from build123d import *

# Parameters (mm, degrees)
F0_R     = 2.26
F0_R_2   = 1.98
F1_DEPTH = 3.17
F2_DEPTH = 7.62
F3_SIZE  = 1.8


with BuildPart() as f1:
    # F0 (on Top) → F1 (new body)
    with BuildSketch(Plane.XY):
        with BuildLine():
            Line((0, -32.255), (0, 0))
            Line((0, 0), (0, 32.255))
            Line((0, 32.255), (-30.1, 32.255))
            ThreePointArc((-30.1, 32.255), (-34.342641, 30.497641), (-36.1, 26.255))
            Line((-36.1, 26.255), (-36.1, -26.255))
            ThreePointArc((-36.1, -26.255), (-34.342641, -30.497641), (-30.1, -32.255))
            Line((-30.1, -32.255), (0, -32.255))
        make_face()
        with Locations((-25.91, -22.225)):
            Circle(F0_R, mode=Mode.SUBTRACT)
        with Locations((-20.32, -26.415)):
            Circle(F0_R_2, mode=Mode.SUBTRACT)
        with Locations((-20.32, -15.855)):
            Circle(F0_R_2, mode=Mode.SUBTRACT)
        with Locations((-20.32, -5.295)):
            Circle(F0_R_2, mode=Mode.SUBTRACT)
        with Locations((-25.91, 0)):
            Circle(F0_R, mode=Mode.SUBTRACT)
        with Locations((-20.32, 5.295)):
            Circle(F0_R_2, mode=Mode.SUBTRACT)
        with Locations((-20.32, 15.855)):
            Circle(F0_R_2, mode=Mode.SUBTRACT)
        with Locations((-25.91, 22.225)):
            Circle(F0_R, mode=Mode.SUBTRACT)
        with Locations((-20.32, 26.415)):
            Circle(F0_R_2, mode=Mode.SUBTRACT)
        with BuildLine():
            Line((-30.1, 32.255), (0, 32.255))
            ThreePointArc((0, 32.255), (-0.743949, 34.051051), (-2.54, 34.795))
            Line((-2.54, 34.795), (-11, 34.795))
            Line((-11, 34.795), (-18.1, 36.32))
            Line((-18.1, 36.32), (-30.1752, 36.32))
            ThreePointArc((-30.1752, 36.32), (-35.77888, 33.99888), (-38.1, 28.3952))
            Line((-38.1, 28.3952), (-38.1, 0))
            Line((-38.1, 0), (-38.1, -28.3952))
            ThreePointArc((-38.1, -28.3952), (-35.77888, -33.99888), (-30.1752, -36.32))
            Line((-30.1752, -36.32), (-18.1, -36.32))
            Line((-18.1, -36.32), (-11, -34.795))
            Line((-11, -34.795), (-2.54, -34.795))
            ThreePointArc((-2.54, -34.795), (-0.743949, -34.051051), (0, -32.255))
            Line((0, -32.255), (-30.1, -32.255))
            ThreePointArc((-30.1, -32.255), (-34.342641, -30.497641), (-36.1, -26.255))
            Line((-36.1, -26.255), (-36.1, 26.255))
            ThreePointArc((-36.1, 26.255), (-34.342641, 30.497641), (-30.1, 32.255))
        make_face()
    extrude(amount=F1_DEPTH)

    # F0 (on Top) → F2 (join)
    with BuildSketch(Plane.XY):
        with BuildLine():
            Line((-30.1, 32.255), (0, 32.255))
            ThreePointArc((0, 32.255), (-0.743949, 34.051051), (-2.54, 34.795))
            Line((-2.54, 34.795), (-11, 34.795))
            Line((-11, 34.795), (-18.1, 36.32))
            Line((-18.1, 36.32), (-30.1752, 36.32))
            ThreePointArc((-30.1752, 36.32), (-35.77888, 33.99888), (-38.1, 28.3952))
            Line((-38.1, 28.3952), (-38.1, 0))
            Line((-38.1, 0), (-38.1, -28.3952))
            ThreePointArc((-38.1, -28.3952), (-35.77888, -33.99888), (-30.1752, -36.32))
            Line((-30.1752, -36.32), (-18.1, -36.32))
            Line((-18.1, -36.32), (-11, -34.795))
            Line((-11, -34.795), (-2.54, -34.795))
            ThreePointArc((-2.54, -34.795), (-0.743949, -34.051051), (0, -32.255))
            Line((0, -32.255), (-30.1, -32.255))
            ThreePointArc((-30.1, -32.255), (-34.342641, -30.497641), (-36.1, -26.255))
            Line((-36.1, -26.255), (-36.1, 26.255))
            ThreePointArc((-36.1, 26.255), (-34.342641, 30.497641), (-30.1, 32.255))
        make_face()
    extrude(amount=F2_DEPTH)

    # F3
    f3_edges = [f1.edges().sort_by_distance(p)[0] for p in [
        (-28.17, -22.225, 3.17),
        (-28.17, 0, 3.17),
        (-28.17, 22.225, 3.17),
    ]]
    chamfer(f3_edges, length=F3_SIZE)


solid = f1.part
Verification items for the finished model (mm, model axes). A direction names the side the tool comes from. Give positions to 0.01 mm unless a question says otherwise; leave off trailing zeros. Write each loop counter-clockwise with the first axis right and the second up, starting at its lowest first coordinate (ties: lowest second). Pieces come first, ordered by that corner, then holes.
(1) Material ranges on line 1 (Y direction, x = -25.91, z = 0.3) (3 decimals); line 2 (Y direction, x = -21, z = 5.5) (3 decimals); line 3 (X direction, y = 19.5, z = 7.25), recorded low to high.
(2) Mould release check, pull along X, two halves, no side actions. Record for faces 4 (the face through (-0.724, 34.031, 3.757)), 5 (the face through (-37, 8, 7.62)), 6 (the face through (-18.43, -4.7, 1.56)): +X half, -X half, draft (parallel to the pull), parting line (faces both ways), or undercut.
(3) Cross-section at C-C (x = -20.32). State how many separate pieces and enclosed holes the cut face has, plus the area to 3 significant figures.
(4) Access from +Z, -Z, +X, -X, +Y, -Y to the whole of each face (thin tool, end or side, straight path). Record for faces 1 (the face through (-18.49, 15.1, 1.56)), 2 (the face through (-15, 32.255, 5)), 3 (the face through (-7, 34.795, 4)).
(5) Cross-section at A-A (x = -25.91). Enter the section's corners in (y, z) (3 decimals).
(6) Gauge pin test, flat ends, axial feed: pin 1 (6.5 mm diameter, centred on x = -20.32, y = -15.855, fed in from +Z); pin 2 (1.3 mm diameter, centred on x = -12.5, z = 4.5, fed in from +Y); pin 3 (6 mm diameter, centred on x = -25.91, y = -22.225, fed in from +Z). Record the tip position at first contact, or that the pin passes through.
(7) Cross-section at B-B (y = 0). Enter the section's corners in (x, z).
Worked out:
1. line 1: y = -36.32 to -24.485, -19.965 to -2.26, 2.26 to 19.965, 24.485 to 36.32
1. line 2: y = -36.32 to -32.255, 32.255 to 36.32
1. line 3: x = -38.1 to -36.1
2. face 4: +X half
2. face 5: draft
2. face 6: undercut
3. separate pieces: 7
3. enclosed holes: 0
3. area: 191 mm2
4. face 1: +Z, -Z
4. face 2: +Z, +X
4. face 3: +Z, -Z, +X, +Y
5. outline: (-36.32, 0) - (-24.485, 0) - (-24.485, 1.37) - (-26.285, 3.17) - (-32.255, 3.17) - (-32.255, 7.62) - (-36.32, 7.62) - close; (-19.965, 0) - (-2.26, 0) - (-2.26, 1.37) - (-4.06, 3.17) - (-18.165, 3.17) - (-19.965, 1.37) - close; (2.26, 0) - (19.965, 0) - (19.965, 1.37) - (18.165, 3.17) - (4.06, 3.17) - (2.26, 1.37) - close; (24.485, 0) - (36.32, 0) - (36.32, 7.62) - (32.255, 7.62) - (32.255, 3.17) - (26.285, 3.17) - (24.485, 1.37) - close
6. pin 1: stops at z = 3.17
6. pin 2: stops at y = 35.26
6. pin 3: stops at z = 2.11
7. outline: (-38.1, 0) - (-28.17, 0) - (-28.17, 1.37) - (-29.97, 3.17) - (-36.1, 3.17) - (-36.1, 7.62) - (-38.1, 7.62) - close; (-23.65, 0) - (0, 0) - (0, 3.17) - (-21.85, 3.17) - (-23.65, 1.37) - close
